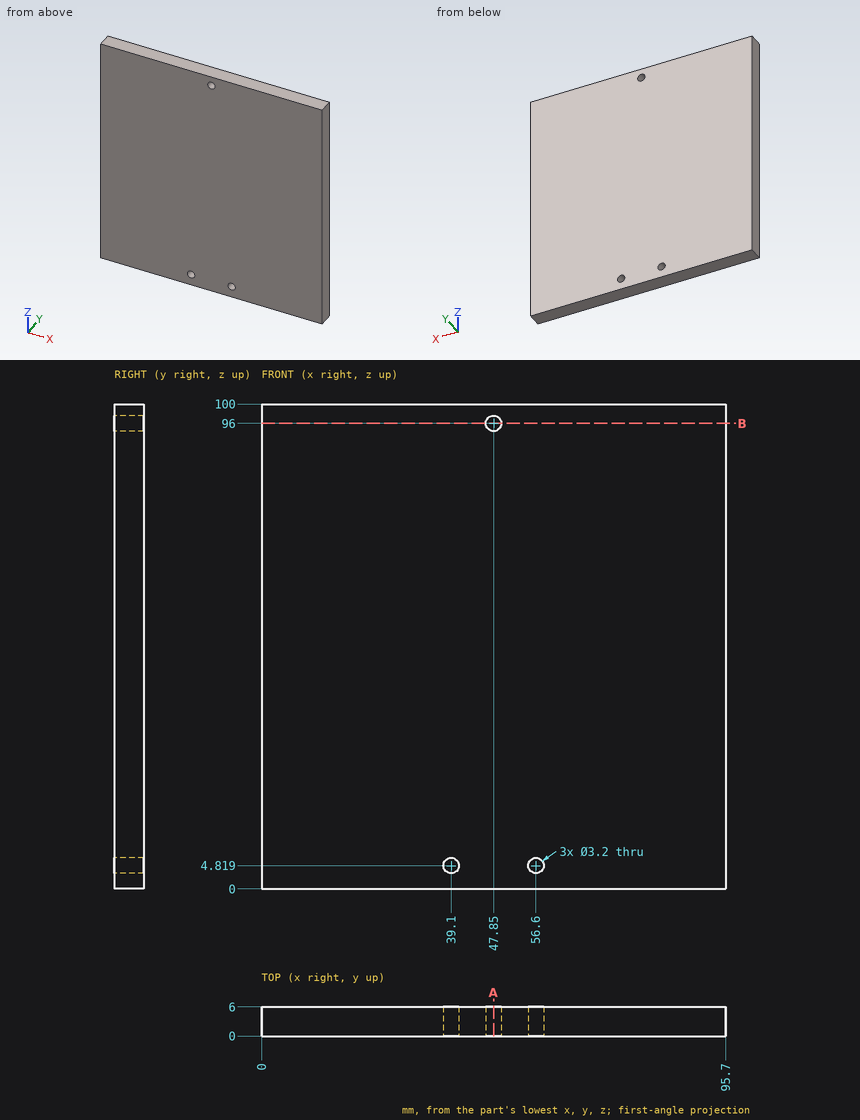
Geometry: see drawing. Coordinates: mm, zero at the bounding-box minimum. Coordinates: 2 decimals unless noted, no trailing zeros. Loops run counter-clockwise (first coordinate to the right, second up) from the corner with the lowest first, then second, coordinate; pieces in that order, holes last. Notation, with made-up numbers: (79.25, 39) - (95.25, 39) arc R32 ccw to (95.25, 73) - close; hole circle Ø9 at (11.25, 85.25). An arc over 180 degrees is marked (long way). Put each result on its own line as item: value. Start each with the question number.
Q1. Cut plane B-B, the plane z = 96. Return loops of the section in (x, y).
Q2. Cut plane A-A, the plane x = 47.85. Return loops of the section in (y, z), and give its area (3 significant figures).
Q3. Line query: line 1 (X direction, y = 1.7, z = 96); line 2 (Z direction, x = 47.85, y = 2.95); line 3 (Z direction, x = 39.1, y = 3.65). Output: solid intervals per line, ascending.
Filled sheet:
1. outline: (0, 0) - (46.25, 0) - (46.25, 6) - (0, 6) - close; (49.45, 0) - (95.7, 0) - (95.7, 6) - (49.45, 6) - close
2. outline: (0, 0) - (6, 0) - (6, 94.4) - (0, 94.4) - close; (0, 97.6) - (6, 97.6) - (6, 100) - (0, 100) - close
2. area: 581 mm²
3. line 1: 0 to 46.25, 49.45 to 95.7
3. line 2: 0 to 94.4, 97.6 to 100
3. line 3: 0 to 3.22, 6.42 to 100
